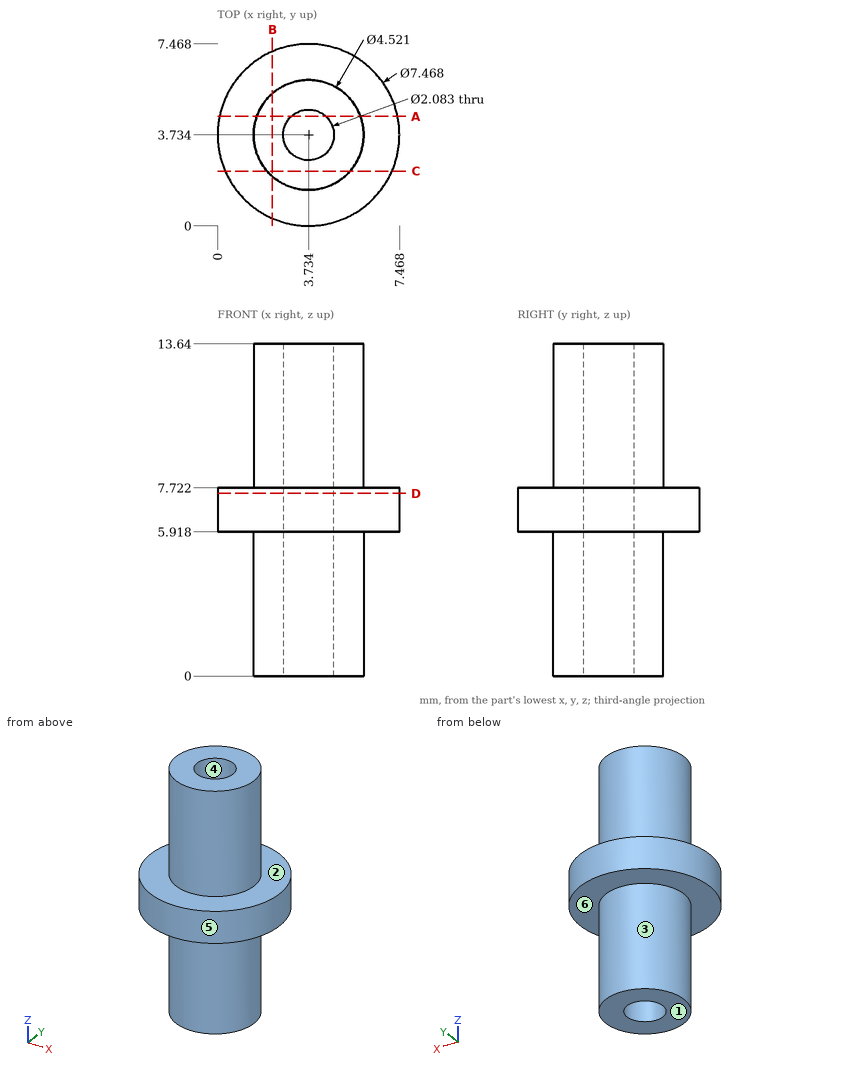
The drawing under review shows one solid part. Ordinate dimensions are in mm from its lowest x, y, z. A direction names the side the tool comes from. Coordinates: 2 decimals unless noted, no trailing zeros. Order: outer loops, then holes, each group sorted by start corner. A loop starts at its lowest first (then second) coordinate and runs counter-clockwise, first axis right, second up. Notation, with made-up numbers: M 34.5,1.5 L 83.5,1.5 A23 cw 83.5,29.5 Z; hole C 49.25,-33 d5. An arc over 180 degrees is marked long. One line per question, with ' | ' between items.
(1) Insertion check: pin 1 (1.2 mm diameter, centred on x = 3.73, y = 3.73, fed in from -Z); pin 2 (4 mm diameter, centred on x = 4.5, z = 2, fed in from +Y); pin 3 (1.5 mm diameter, centred on x = 2.5, z = 2, fed in from -Y) (1 decimal). Each pin has a flat end and moves straight along its axis. Give the tip position at first contact, or say it passes through.
Geometry results:
pin 1: passes through | pin 2: stops at y = 5.99 | pin 3: stops at y = 1.5
(2) Machinability: for the marked faces 1, 2 and 3, which of the approach directions +Z, -Z, +X, -X, +Y, -Y give a long, thin tool a straight path to every point of the face, cutting with its end or side? Answer none if there is none.
Geometry results:
face 1: -Z, +X, -X, +Y, -Y | face 2: +Z | face 3: -Z
(3) Add section A-A, the plane y = 4.5. Write out the cut boundary in (x, z).
Geometry results:
outline: M 0.08,5.92 L 1.61,5.92 L 1.61,0 L 3.03,0 L 3.03,13.64 L 1.61,13.64 L 1.61,7.72 L 0.08,7.72 Z; M 4.44,0 L 5.86,0 L 5.86,5.92 L 7.39,5.92 L 7.39,7.72 L 5.86,7.72 L 5.86,13.64 L 4.44,13.64 Z
(4) Add section D-D, the plane z = 7.5. Write out the cut boundary in (x, y) (1 decimal).
Geometry results:
outline: C 3.7,3.7 d7.5; hole C 3.7,3.7 d2.1
(5) The part is to be moulded in two halves that separate along X. For the marked faces 4, 5 and 6, say which applies: +X half, -X half, draft (parallel to the pull), parting line (faces both ways), or undercut.
Geometry results:
face 4: undercut | face 5: parting line | face 6: draft
(6) For probe 1 along Y at (x, z) = (3.75, 9.25) (1 decimal); probe 2 along Y at (x, z) = (4.5, 8) (1 decimal); probe 3 along Z at (x, y) = (5.75, 6.5), list the stretches that pass through material, from the lowest coordinate up. Write a range as from..to.
Geometry results:
probe 1: y = 1.5..2.7, 4.8..6 | probe 2: y = 1.6..3, 4.4..5.9 | probe 3: z = 5.92..7.72
(7) Add section B-B, the plane x = 2.25. Write out the cut boundary in (y, z).
Geometry results:
outline: M 0.31,5.92 L 2.03,5.92 L 2.03,0 L 5.44,0 L 5.44,5.92 L 7.16,5.92 L 7.16,7.72 L 5.44,7.72 L 5.44,13.64 L 2.03,13.64 L 2.03,7.72 L 0.31,7.72 Z
